Autodesk Inventor part; units mm, degrees
ref_plane "YZ Plane" through (0, 0, 0) normal (1, 0, 0) x (0, 1, 0)
ref_plane "XZ Plane" through (0, 0, 0) normal (0, 1, 0) x (-1, 0, 0)
ref_plane "XY Plane" through (0, 0, 0) normal (0, 0, 1) x (1, 0, 0)
sketch "Sketch1" plane through (0, 0, 0) normal (0, 1, 0) x (-1, 0, 0)
  line L0 (0, 6.35) -> (0, -6.35) construction
  line L1 (0, 0) -> (-6.35, 0) construction
  line L2 (0, -6.35) -> (0, -44.45) construction
  line L3 (0, -44.45) -> (12.7, -44.45) construction
  line L4 (0, -44.45) -> (0, -69.85) construction
  line L5 (-6.35, 0) -> (-12.7, 0) construction
  line L6 (0, 6.35) -> (0, 31.75) construction
  circle A0 centre (0, 31.75) radius 2.4892 construction
  circle A1 centre (0, 19.05) radius 2.4892
  circle A2 centre (0, 6.35) radius 2.4892 construction
  circle A3 centre (0, -6.35) radius 2.4892 construction
  circle A4 centre (0, -19.05) radius 2.4892
  circle A5 centre (0, -31.75) radius 2.4892 construction
  circle A6 centre (0, -44.45) radius 2.4892
  circle A7 centre (0, -57.15) radius 2.4892 construction
  circle A8 centre (0, -69.85) radius 2.4892
  circle A9 centre (12.7, -44.45) radius 2.4892 construction
  line L7 (12.7, -44.45) -> (38.1, -44.45) construction
  circle A10 centre (25.4, -44.45) radius 2.4892
  circle A11 centre (38.1, -44.45) radius 2.4892 construction
  line L8 (12.7, 31.75) -> (-12.7, 31.75)
  line L9 (12.7, 31.75) -> (12.7, -31.75)
  line L10 (12.7, -31.75) -> (38.1, -31.75)
  line L11 (38.1, -31.75) -> (38.1, -57.15)
  line L12 (38.1, -57.15) -> (12.7, -57.15)
  line L13 (12.7, -57.15) -> (12.7, -82.55)
  line L14 (12.7, -82.55) -> (-12.7, -82.55)
  line L15 (-12.7, -82.55) -> (-12.7, -12.7)
  line L16 (-12.7, -12.7) -> (-25.4, -12.7)
  line L17 (-25.4, -12.7) -> (-25.4, 12.7) construction
  line L18 (-25.4, 12.7) -> (-12.7, 12.7)
  line L19 (-12.7, 12.7) -> (-12.7, 31.75)
  circle A12 centre (-25.4, 0) radius 2.4892
  line L20 (-25.4, 12.7) -> (-38.1, 12.7)
  line L21 (-38.1, 12.7) -> (-38.1, -12.7)
  line L22 (-38.1, -12.7) -> (-25.4, -12.7)
  point P0 (0, 31.75)
  point P1 (0, -82.55)
  dimension "d0" = 12.7
  dimension "d1" = 6.35
  dimension "d2" = 38.1
  dimension "d3" = 12.7
  dimension "d4" = 25.4
  dimension "d6" = 25.4
  dimension "d15" = 4.9784
  dimension "d18" = 12.7
  dimension "d23" = 4.9784
  dimension "d24" = 25.4
  dimension "d27" = 12.7
  dimension "d32" = 25.4
  dimension "d33" = 12.7
  dimension "d34" = 12.7
  dimension "d36" = 12.7
  dimension "d40" = 4.9784
  dimension "d41" = 12.7
extrude "Extrusion1" add sketch "Sketch1" along normal blind 6.35
fillet "Fillet1" radius 6.35 12 edges at (-12.7, 3.175, 31.75) (12.7, 3.175, 31.75) (12.7, 3.175, 12.7) (-12.7, 3.175, -31.75) (-38.1, 3.175, -31.75) (-38.1, 3.175, -57.15) (-12.7, 3.175, -57.15) (-12.7, 3.175, -82.55) (12.7, 3.175, -82.55) (12.7, 3.175, -12.7) (38.1, 3.175, 12.7) (38.1, 3.175, -12.7)
properties part number "STRU_021_DVBSBracket2" material "Aluminum 6061"
Design review of the part built by this model. Coordinates are the model's own, in mm. A direction names the side the tool comes from. Coordinates: 2 decimals unless noted, no trailing zeros. Loops run counter-clockwise (first coordinate to the right, second up) from the corner with the lowest first, then second, coordinate; pieces in that order, holes last.
Q1. We need section A-A on x = 25.4. State the section outline as (y, z) points.
Reported:
outline: (0, -12.7) - (6.35, -12.7) - (6.35, -2.49) - (0, -2.49) - close; (0, 2.49) - (6.35, 2.49) - (6.35, 12.7) - (0, 12.7) - close
Q2. We need section B-B on z = -69.85. State the section outline as (x, y) points, and give its area (3 significant figures).
Reported:
outline: (-12.7, 0) - (-2.49, 0) - (-2.49, 6.35) - (-12.7, 6.35) - close; (2.49, 0) - (12.7, 0) - (12.7, 6.35) - (2.49, 6.35) - close
area: 130 mm2
Q3. For pin 1 (3 mm diameter, centred on x = 19.5, y = 3.5, fed in from +Z); pin 2 (3 mm diameter, centred on y = 2, z = 9, fed in from -X); pin 3 (1.9 mm diameter, centred on y = 2.5, z = -57.5, fed in from +X), all flat-tipped, find the tip position at first contact; note any pin that passes through.
Reported:
pin 1: stops at z = 12.79
pin 2: stops at x = -12.7
pin 3: stops at x = 12.7
Q4. Tool access review of faces 4 (the face through (-25, 3, -57.15)), 5 (the face through (0.54, 3.13, -42.02)), 6 (the face through (12.7, 3, 22)), 7 (the face through (25, 3, -12.7)): name each direction out of +Z, -Z, +X, -X, +Y, -Y from which nothing blocks a thin tool from reaching the whole face with its end or side.
Reported:
face 4: -Z, -X, +Y, -Y
face 5: +Y, -Y
face 6: +Z, +X, +Y, -Y
face 7: -Z, +X, +Y, -Y
Q5. We need section D-D on x = -14. State the section outline as (y, z) points, and give its area (3 significant figures).
Reported:
outline: (0, -59.65) - (6.35, -59.65) - (6.35, -29.25) - (0, -29.25) - close
area: 193 mm2
Q6. The part is to be moulded in two halves that separate along Z. For faces 1 (the face through (1, 0, -25)), 2 (the face through (36.19, 3.22, 10.89)), 3 (the face through (-24.86, 3.13, -42.02)), say which applies: +Z half, -Z half, draft (parallel to the pull), parting line (faces both ways), or undercut.
Reported:
face 1: draft
face 2: +Z half
face 3: undercut
Q7. We need section C-C on y = 2. State how many separate pieces and enclosed holes the cut face has, and give its area (3 significant figures).
Reported:
separate pieces: 1
enclosed holes: 6
area: 4,040 mm2
Q8. To check wall thickness, follow line 1 (Z direction, x = 0, y = 2.5); line 2 (X direction, y = 3, z = -46); line 3 (Z direction, x = 25.4, y = 4.5). State the ranges of each line that lie inside material, in increasing order.
Reported:
line 1: z = -82.55 to -72.34, -67.36 to -46.94, -41.96 to -21.54, -16.56 to 16.56, 21.54 to 31.75
line 2: x = -38.1 to -27.35, -23.45 to -1.95, 1.95 to 12.7
line 3: z = -12.7 to -2.49, 2.49 to 12.7
